from build123d import *

# Parameters (mm, degrees)
F0_W     = 29.21
F0_H     = 46.355
F1_DEPTH = 2.54
F0_H_2   = 4.445
F0_W_2   = 0.635
F2_DEPTH = 6.35


with BuildPart() as f1:
    # F0 (on Front) → F1 (new body)
    with BuildSketch(Plane.XZ):
        with Locations((0, 2.2225)):
            Rectangle(F0_W, F0_H)
    extrude(amount=F1_DEPTH)

    # F0 (on Front) → F2 (join)
    with BuildSketch(Plane.XZ):
        with Locations((0, -23.1775)):
            Rectangle(F0_W, F0_H_2)
        with Locations((14.9225, -23.1775)):
            Rectangle(F0_W_2, F0_H_2)
        with Locations((-14.9225, 2.2225)):
            Rectangle(F0_W_2, F0_H)
        with Locations((-15.5575, 2.2225)):
            Rectangle(F0_W_2, F0_H)
        with Locations((-15.5575, -23.1775)):
            Rectangle(F0_W_2, F0_H_2)
        with Locations((-14.9225, -23.1775)):
            Rectangle(F0_W_2, F0_H_2)
        Polygon((15.875, -25.4), (15.24, -25.4), (14.605, -25.4), (-14.605, -25.4), (-15.24, -25.4), (-15.875, -25.4), (-15.875, -29.845), (15.875, -29.845), align=None)
        with Locations((15.5575, -23.1775)):
            Rectangle(F0_W_2, F0_H_2)
        with Locations((15.5575, 2.2225)):
            Rectangle(F0_W_2, F0_H)
        with Locations((14.9225, 2.2225)):
            Rectangle(F0_W_2, F0_H)
    extrude(amount=F2_DEPTH)


solid = f1.part
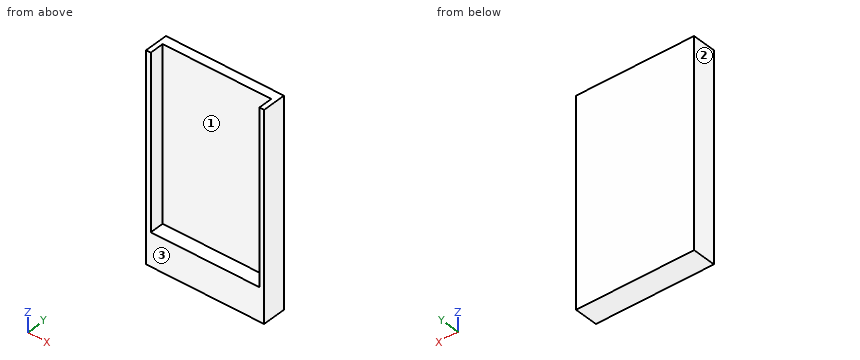
For this review, take the finished solid that the model builds, in its own axes (mm). Face numbers are marked on the shaded views. Coordinates: 2 decimals unless noted, no trailing zeros. Loops run counter-clockwise (first coordinate to the right, second up) from the corner with the lowest first, then second, coordinate; pieces in that order, holes last. Notation, with made-up numbers: (47, 41.5) - (99, 41.5) arc R24 ccw to (99, 66.5) - close; hole circle Ø4 at (14, 89.25). An arc over 180 degrees is marked (long way). Use a Markdown table: item, result. Add a question column.
Item 1: For line 1 (X direction, y = -4.5, z = 20) (3 decimals); line 2 (Y direction, x = 0, z = 13.5); line 3 (Z direction, x = 13, y = -5) (3 decimals), list the stretches that pass through material, from the lowest coordinate up.
Item 2: We need section B-B (y = -4). Give the boundary of the cut face in (x, z) (3 decimals).
Item 3: We need section C-C (x = 13). Give the boundary of the cut face in (y, z) (3 decimals), and give its area (3 significant figures).
Item 4: Mouldability with a two-part tool opening along X and no side actions: class the marked faces 1, 2 and 3 as pulls with the +X half, pulls with the -X half, needs draft (parallel to the pull), parting line crosses it, or undercut.
Item 5: We need section A-A (z = 10). Give the boundary of the cut face in (x, y) (3 decimals).
Item 6: Insertion check: pin 1 Ø14.5 at (x, z) = (-3, 12) entering from -Y. The pin has a flat end and moves straight along its axis. Give the tip position at first contact, or say it passes through.
Results list:
| question | item | result |
|---|---|---|
| 1 | line 1 | x = -15.875 to -14.605, 14.605 to 15.875 |
| 1 | line 2 | y = -2.54 to 0 |
| 1 | line 3 | z = -29.845 to -20.955 |
| 2 | outline | (-15.875, -29.845) - (15.875, -29.845) - (15.875, 25.4) - (14.605, 25.4) - (14.605, -20.955) - (-14.605, -20.955) - (-14.605, 25.4) - (-15.875, 25.4) - close |
| 3 | outline | (-6.35, -29.845) - (0, -29.845) - (0, 25.4) - (-2.54, 25.4) - (-2.54, -20.955) - (-6.35, -20.955) - close |
| 3 | area | 174 mm^2 |
| 4 | face 1 | undercut |
| 4 | face 2 | pulls with the -X half |
| 4 | face 3 | needs draft |
| 5 | outline | (-15.875, -6.35) - (-14.605, -6.35) - (-14.605, -2.54) - (14.605, -2.54) - (14.605, -6.35) - (15.875, -6.35) - (15.875, 0) - (-15.875, 0) - close |
| 6 | pin 1 | stops at y = -2.54 |
